Answer from the drawing. Dimensions are ordinates in mm from the lowest x, y and z of the part. Give positions to 0.01 mm unless a question says otherwise; leave off trailing zeros. Loops run counter-clockwise (first coordinate to the right, second up) from the corner with the lowest first, then second, coordinate; pieces in that order, holes last. Notation, with made-up numbers: (25, 14) - (71, 14) arc R25 ccw to (71, 52) - close; hole circle Ø1 at (49, 39.5). An arc over 180 degrees is marked (long way). One line per question, with ' | ' between items. Start each with the question number.
1. Find the intervals of material crossed by line 1 (X direction, y = 1.5, z = 12); line 2 (Z direction, x = 107.95, y = 2.25); line 3 (X direction, y = 0.9, z = 22.75), in increasing order.
2. Section C-C (z = 5.25) is taken. Determine the outline of the cut face in (x, y) (3 decimals).
3. Section B-B (z = 20) is taken. Determine the outline of the cut face in (x, y) (3 decimals).
4. Section A-A (y = 2.55) is taken. Determine the outline of the cut face in (x, z).
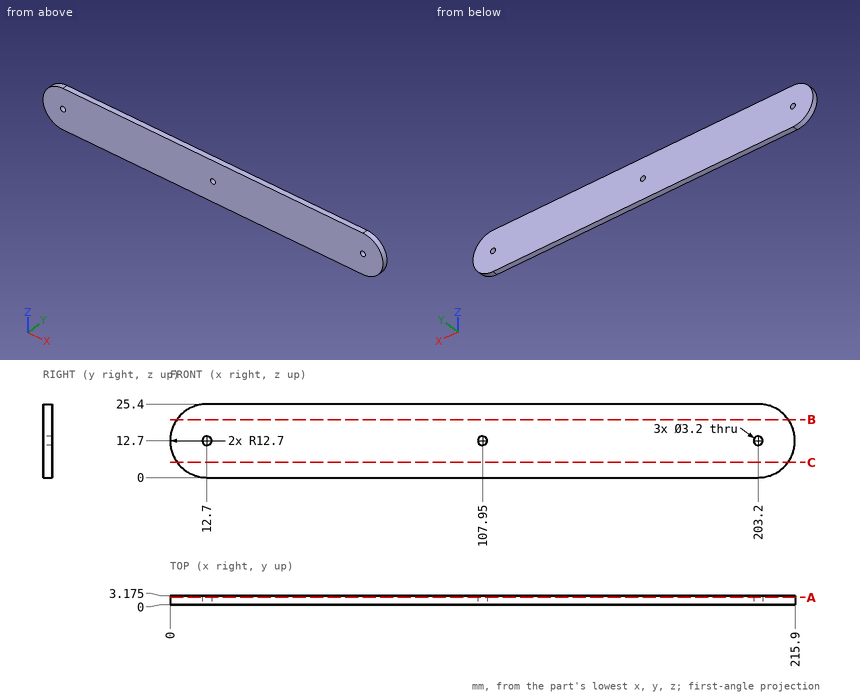
Conclusion:
1) line 1: 0.02 to 11.26, 14.14 to 106.51, 109.39 to 201.76, 204.64 to 215.88 | line 2: 0 to 11.1, 14.3 to 25.4 | line 3: 4.94 to 210.96
2) outline: (2.415, 0) - (213.485, 0) - (213.485, 3.175) - (2.415, 3.175) - close
3) outline: (2.308, 0) - (213.592, 0) - (213.592, 3.175) - (2.308, 3.175) - close
4) outline: (12.7, 0) - (203.2, 0) arc R12.7 ccw to (203.2, 25.4) - (12.7, 25.4) arc R12.7 ccw to start; hole circle Ø3.2 at (12.7, 12.7); hole circle Ø3.2 at (107.95, 12.7); hole circle Ø3.2 at (203.2, 12.7)
